The figure shows three views and two pictorial views of one solid part (mm, origin at its lowest corner). Answer the questions. A direction names the side the tool comes from. Give positions to 0.01 mm unless a question says otherwise; leave off trailing zeros. Write each loop counter-clockwise with the first axis right and the second up, starting at its lowest first coordinate (ties: lowest second). Pieces come first, ordered by that corner, then holes. Notation, with made-up numbers: M 78,39.25 L 132,39.25 A10 ccw 132,43.25 Z; hole C 58,-35.75 d3. An arc over 180 degrees is marked long. Return JSON: item names as keys, results as strings.
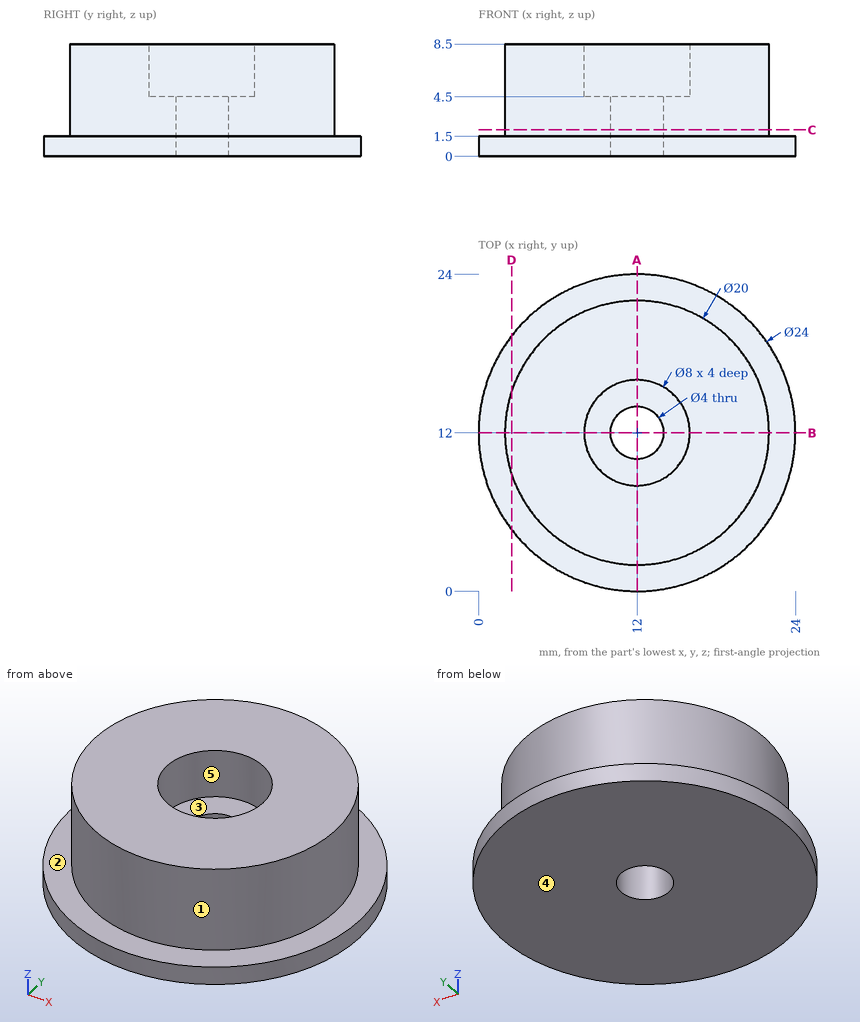
Item 1: A cutting plane is placed at A-A, the plane x = 12. Write down the section's boundary in (y, z), plus the area to 3 significant figures.
Geometry results:
{"outline": "M 0,0 L 10,0 L 10,4.5 L 8,4.5 L 8,8.5 L 2,8.5 L 2,1.5 L 0,1.5 Z; M 14,0 L 24,0 L 24,1.5 L 22,1.5 L 22,8.5 L 16,8.5 L 16,4.5 L 14,4.5 Z", "area": "126 mm2"}
Item 2: Determine the mould class of the marked faces 1, 2 and 3 for opening direction X: +X half, -X half, draft (parallel to the pull), parting line (faces both ways), or undercut.
Geometry results:
{"face 1": "parting line", "face 2": "draft", "face 3": "undercut"}
Item 3: Which of the six approach directions +Z, -Z, +X, -X, +Y, -Y give full straight-line access (tool end or side, diameter ignored) to the marked faces 4 and 5?
Geometry results:
{"face 4": "-Z, +X, -X, +Y, -Y", "face 5": "+Z"}
Item 4: Given pin 1 Ø1 at (x, z) = (6.5, 3.5) entering from +Y; pin 2 Ø4 at (x, y) = (13, 13.5) entering from +Z; pin 3 Ø3 at (y, z) = (13, 7.5) entering from +X, each flat-ended and moving along its own axis, determine where each tip first touches the part or whether it passes through.
Geometry results:
{"pin 1": "stops at y = 20.66", "pin 2": "stops at z = 4.5", "pin 3": "stops at x = 22"}
Item 5: A cutting plane is placed at D-D, the plane x = 2.5. Write down the section's boundary in (y, z).
Geometry results:
{"outline": "M 4.67,0 L 19.33,0 L 19.33,1.5 L 15.12,1.5 L 15.12,8.5 L 8.88,8.5 L 8.88,1.5 L 4.67,1.5 Z"}
Item 6: A cutting plane is placed at C-C, the plane z = 2. Write down the section's boundary in (x, y), plus the area to 3 significant figures.
Geometry results:
{"outline": "C 12,12 d20; hole C 12,12 d4", "area": "302 mm2"}
Item 7: Find the intervals of material crossed by line 1 (Y direction, x = 12, z = 2.55); line 2 (Y direction, x = 12, z = 1.35); line 3 (Z direction, x = 3, y = 16.5), in increasing order.
Geometry results:
{"line 1": "y = 2 to 10, 14 to 22", "line 2": "y = 0 to 10, 14 to 24", "line 3": "z = 0 to 1.5"}
